```python
from build123d import *

# Parameters (mm, degrees)
F2_R     = 9.54913
F3_DEPTH = 60.326


with BuildPart() as f1:
    # F0 (on Right) → F1 (revolve)
    with BuildSketch(Plane.YZ):
        Polygon((0, 19.15033), (0, 0), (63.5, 0), (62.302494, 3.9497), (59.635494, 3.9497), (22.27326, 12.55014), (19.09826, 12.55014), (19.09826, 49.95037), (3.175, 49.95037), (3.175, 19.15033), align=None)
    revolve(axis=Axis((0, 4.994582, -26.29916), (0, 1, 0)))

    # F2 (on face) → F3 (cut, through all)
    with BuildSketch(Plane.XZ.offset(-3.175)):
        with Locations((0, 36.885909)):
            Circle(F2_R)
        with Locations((63.185069, -26.29916)):
            Circle(F2_R)
        with Locations((0, -89.484229)):
            Circle(F2_R)
        with Locations((-63.185069, -26.29916)):
            Circle(F2_R)
    extrude(amount=-F3_DEPTH, mode=Mode.SUBTRACT)


solid = f1.part
```
Here's how the part is built. I have some questions about the finished solid (model axes, mm). A direction names the side the tool comes from. Coordinates: 2 decimals unless noted, no trailing zeros. Order: outer loops, then holes, each group sorted by start corner. A loop starts at its lowest first (then second) coordinate and runs counter-clockwise, first axis right, second up.
1) I need wall thicknesses on line 1 (X direction, y = 9.5, z = -21); line 2 (Z direction, x = 65.5, y = 10.5); line 3 (X direction, y = 6.5, z = -39.5). Which ranges of each line are inside material? Lowest first, please.
2) Imagine slicing it at A-A on x = 0. List the corners of the cut face in (y, z) for me (1 decimal).
3) Imagine slicing it at D-D on z = 25.5. List the corners of the cut face in (x, y) for me (3 decimals), and give its area (3 significant figures).
4) We'd pull the mould along X, two halves only. Please class faces 4 (the face through (7.974, 63.425, -0.979)), 5 (the face through (-7.04, 11.03, -83.03)), 6 (the face through (18, 19.098, 9)): +X half, -X half, draft (parallel to the pull), parting line (faces both ways), or undercut.
5) Which directions (+Z, -Z, +X, -X, +Y, -Y) give clear straight access to the entire face, cutting with the end or side of a thin tool? Please do faces 1 (the face through (-16, 32.19, -47.17)), 2 (the face through (-23.64, 20.66, -57.13)), 3 (the face through (-33, 3.175, 7)).
6) Imagine slicing it at C-C on y = 6. List the corners of the cut face in (x, z) for me, and give its area (3 significant figures).
7) Imagine slicing it at B-B on x = -65.5. List the corners of the cut face in (y, z) for me (3 decimals).
8) Will these pins go through, and if not, where does the flat tip stop? pin 1 (25 mm diameter, centred on x = 0, z = -89.48, fed in from +Y); pin 2 (25 mm diameter, centred on x = 63.19, z = -26.3, fed in from -Y) (3 decimals); pin 3 (2 mm diameter, centred on x = -13, y = 51, fed in from +Z); pin 4 (15.5 mm diameter, centred on x = -63.19, z = -26.3, fed in from +Y).
Response values:
1. line 1: x = -76.07 to -71.13, -55.24 to -25.76, 25.76 to 55.24, 71.13 to 76.07
1. line 2: z = -65.33 to -35.56, -17.03 to 12.74
1. line 3: x = -75.1 to -22.75, 22.75 to 75.1
2. outline: (0, -71.7) - (3.2, -71.7) - (3.2, -79.9) - (19.1, -79.9) - (19.1, -65.1) - (22.3, -65.1) - (59.6, -56.5) - (62.3, -56.5) - (63.5, -52.6) - (0, -52.6) - close; (0, 0) - (63.5, 0) - (62.3, 3.9) - (59.6, 3.9) - (22.3, 12.6) - (19.1, 12.6) - (19.1, 27.3) - (3.2, 27.3) - (3.2, 19.2) - (0, 19.2) - close; (3.2, -102.5) - (19.1, -102.5) - (19.1, -99) - (3.2, -99) - close; (3.2, 46.4) - (19.1, 46.4) - (19.1, 50) - (3.2, 50) - close
3. outline: (-55.954, 3.175) - (55.954, 3.175) - (55.954, 19.098) - (-55.954, 19.098) - close
3. area: 1,780 mm2
4. face 4: parting line
4. face 5: undercut
4. face 6: draft
5. face 1: +Y, -Y
5. face 2: +Y
5. face 3: -Y
6. outline: circle Ø152.5 at (0, -26.3); hole circle Ø19.1 at (-63.19, -26.3); hole circle Ø52.6 at (0, -26.3); hole circle Ø19.1 at (0, -89.48); hole circle Ø19.1 at (0, 36.89); hole circle Ø19.1 at (63.19, -26.3)
6. area: 14,900 mm2
7. outline: (3.175, -65.334) - (19.098, -65.334) - (19.098, -35.563) - (3.175, -35.563) - close; (3.175, -17.035) - (19.098, -17.035) - (19.098, 12.736) - (3.175, 12.736) - close
8. pin 1: stops at y = 19.1
8. pin 2: stops at y = 3.175
8. pin 3: stops at z = 3.69
8. pin 4: passes through
